Build history of the part. All positions in model axes, mm. A direction names the side the tool comes from. Round coordinates to 2 decimals unless told otherwise and drop trailing zeros. Order: outer loops, then holes, each group sorted by start corner. A loop starts at its lowest first (then second) coordinate and runs counter-clockwise, first axis right, second up. Notation, with made-up numbers: M -39.75,17 L 5.25,17 A13 cw 5.25,22 Z; hole C -6.5,-24 d3. An arc over 180 degrees is marked long. One line per item, written item: value. Start each with the question number.
Item 1: Two-plate mould, pull along Z, no slides. Class faces 5 (the cylindrical face through (-3.417, 24.479, -0.759)), 6 (the flat face through (0, 13, 3)), 7 (the flat face through (0, 13, -3)), 8 (the flat face through (-3.3, 3, 2.2)): +Z half, -Z half, draft (parallel to the pull), parting line (faces both ways), or undercut.
Item 2: Probe L1, parallel to Y at x = 4.5, z = 2; L2, parallel to Y at x = 2.5, z = -1; L3, parallel to Z at x = -3, y = 7. List the from-to ranges inside material, lowest first.
Item 3: Pin check, flat tips, straight feed: pin 1 (1 mm diameter, centred on x = -3, y = 20, fed in from +Z); pin 2 (1 mm diameter, centred on x = 1.5, y = 20.5, fed in from -Z); pin 3 (1.5 mm diameter, centred on y = 5.5, z = -4, fed in from +X). Stop position of each tip, or through.
Item 4: Band-saw the part on B-B, the plane x = 0. Write the cut outline in (y, z).
Item 5: Band-saw the part on A-A, the plane z = 0. Write the cut outline in (x, y).
Item 6: Tool access for faces 1 (the flat face through (-3.3, 23, 2.2)), 2 (the cylindrical face through (-3.417, 1.479, -0.759)), 3 (the flat face through (0, 26, 0)), 4 (the flat face through (0, 20.5, 0)): list every direction of +Z, -Z, +X, -X, +Y, -Y with a clear straight run to the whole face (end or side of a thin tool).
Item 7: Band-saw the part on C-C, the plane x = -4.5. Write the cut outline in (y, z), then the cut area to 3 significant figures.
Item 8: Band-saw the part on D-D, the plane y = 18. Write the cut outline in (x, z).
```python
from build123d import *

# Parameters (mm, degrees)
CROQUIS1_R                 = 3.5
SALIENTE_EXTRUIR1_DEPTH    = 3
CROQUIS2_R                 = 5
SALIENTE_EXTRUIR2_DEPTH    = 20
CROQUIS3_R                 = 3.5
SALIENTE_EXTRUIR3_DEPTH    = 3
CORTAR_EXTRUIR1_DEPTH      = 10
CORTAR_EXTRUIR1_DEPTH_BACK = 11
CROQUIS4_W                 = 6
CROQUIS4_H                 = 15


with BuildPart() as part:
    # Croquis1 → Saliente-Extruir1 (new body)
    with BuildSketch(Plane(origin=(0, 0, 0), x_dir=(1, 0, 0), z_dir=(0, 1, 0))):
        with Locations(Location((0, 0, 0), (0, 0, 270))):
            Circle(CROQUIS1_R)
    extrude(amount=SALIENTE_EXTRUIR1_DEPTH)

    # Croquis2 → Saliente-Extruir2 (add)
    with BuildSketch(Plane(origin=(0, 3, 0), x_dir=(1, 0, 0), z_dir=(0, 1, 0))):
        with Locations(Location((0, 0, 0), (0, 0, 270))):
            Circle(CROQUIS2_R)
    extrude(amount=SALIENTE_EXTRUIR2_DEPTH)

    # Croquis3 → Saliente-Extruir3 (add)
    with BuildSketch(Plane(origin=(0, 23, 0), x_dir=(1, 0, 0), z_dir=(0, 1, 0))):
        with Locations(Location((0, 0, 0), (0, 0, 270))):
            Circle(CROQUIS3_R)
    extrude(amount=SALIENTE_EXTRUIR3_DEPTH)

    # Croquis4 → Cortar-Extruir1 (cut, two sides: drawn at the far end of the back side and taken through both)
    with BuildSketch(Plane(origin=(0, 0, 0), x_dir=(0, 0, -1), z_dir=(1, 0, 0)).offset(-CORTAR_EXTRUIR1_DEPTH_BACK)):
        with Locations((0, 13)):
            Rectangle(CROQUIS4_W, CROQUIS4_H)
    extrude(amount=CORTAR_EXTRUIR1_DEPTH + CORTAR_EXTRUIR1_DEPTH_BACK, mode=Mode.SUBTRACT)


solid = part.part
```
Output:
1. face 5: parting line
1. face 6: undercut
1. face 7: undercut
1. face 8: draft
2. L1: y = 3 to 5.5, 20.5 to 23
2. L2: y = 0 to 5.5, 20.5 to 26
2. L3: z = -4 to -3, 3 to 4
3. pin 1: stops at z = 4.33
3. pin 2: stops at z = -4.9
3. pin 3: stops at x = 3.8
4. outline: M 0,-3.5 L 3,-3.5 L 3,-5 L 23,-5 L 23,-3.5 L 26,-3.5 L 26,3.5 L 23,3.5 L 23,5 L 3,5 L 3,3.5 L 0,3.5 Z; hole M 5.5,-3 L 20.5,-3 L 20.5,3 L 5.5,3 Z
5. outline: M -5,3 L -3.5,3 L -3.5,0 L 3.5,0 L 3.5,3 L 5,3 L 5,5.5 L -5,5.5 Z; M -5,20.5 L 5,20.5 L 5,23 L 3.5,23 L 3.5,26 L -3.5,26 L -3.5,23 L -5,23 Z
6. face 1: +Y
6. face 2: -Y
6. face 3: +Z, -Z, +X, -X, +Y
6. face 4: +X, -X
7. outline: M 3,-2.18 L 5.5,-2.18 L 5.5,2.18 L 3,2.18 Z; M 20.5,-2.18 L 23,-2.18 L 23,2.18 L 20.5,2.18 Z
7. area: 21.8 mm²
8. outline: M -4,-3 A5 ccw 4,-3 Z; M -4,3 L 4,3 A5 ccw Z
